Read the model definition and answer for the solid it produces. Units are mm, in the model's axes. A direction names the side the tool comes from. Round coordinates to 2 decimals unless told otherwise and drop trailing zeros. Loops run counter-clockwise (first coordinate to the right, second up) from the corner with the lowest first, then second, coordinate; pieces in that order, holes last. Notation, with made-up numbers: M -9,-13 L 19,-13 A27 cw 19,15 Z; hole C 73.5,7 d2. An arc over 180 degrees is marked long. Write each question's results on one line, items separated by ' | '.
from build123d import *

# Parameters (mm, degrees)
BULK_DEPTH              = 2.75
BULK_DEPTH_BACK         = 2.8
PEG_BASE_SKETCH_W       = 0.25
PEG_BASE_SKETCH_H       = 0.9
PEGS_DEPTH              = 3.35
RECEPTACLE_DEPTH        = 3.75
RECEPTACLE_DEPTH_BACK   = 0.75
SKETCH3_W               = 0.6
SKETCH3_H               = 0.4
UPPER_FINS_DEPTH        = 0.31
ALTIUM_AXIS_ALIGN_ANGLE = 90


with BuildPart() as part:
    # Base sketch → Bulk (new body, two sides)
    with BuildSketch(Plane.XY) as bulk_sk:
        Polygon((3.7, 2.35), (-3.7, 2.35), (-3.7, 0.896446609), (-2.803553391, 0), (2.803553391, 0), (3.7, 0.896446609), align=None)
    extrude(amount=BULK_DEPTH)
    extrude(bulk_sk.sketch, amount=-BULK_DEPTH_BACK)

    # Peg base sketch → Pegs (add)
    with BuildSketch(Plane(origin=(0, 2.35, 0), x_dir=(1, 0, 0), z_dir=(0, 1, 0))):
        with Locations((3.575, 0)):
            Rectangle(PEG_BASE_SKETCH_W, PEG_BASE_SKETCH_H)
        with Locations((-3.575, 0)):
            Rectangle(PEG_BASE_SKETCH_W, PEG_BASE_SKETCH_H)
    extrude(amount=-PEGS_DEPTH)

    # Base sketch<3> → Receptacle (cut, two sides)
    with BuildSketch(Plane.XY) as receptacle_sk:
        Polygon((-3.45, 1), (-2.7, 0.25), (2.7, 0.25), (3.45, 1), (3.45, 2.1), (-3.45, 2.1), align=None)
    extrude(amount=RECEPTACLE_DEPTH, mode=Mode.SUBTRACT)
    extrude(receptacle_sk.sketch, amount=-RECEPTACLE_DEPTH_BACK, mode=Mode.SUBTRACT)

    # Sketch3 → Upper fins (add)
    with BuildSketch(Plane(origin=(0, 2.35, 0), x_dir=(1, 0, 0), z_dir=(0, 1, 0))):
        with Locations((-2.375, -1.4)):
            Rectangle(SKETCH3_W, SKETCH3_H)
        with Locations((2.375, -1.4)):
            Rectangle(SKETCH3_W, SKETCH3_H)
    extrude(amount=UPPER_FINS_DEPTH)


with BuildPart() as part_1:
    # Altium axis align: moved
    add(part.part.rotate(Axis((0, 0, 0), (1, 0, 0)), ALTIUM_AXIS_ALIGN_ANGLE))


solid = part_1.part
Item 1: A flat-ended cylindrical pin translates along its axis: pin 1 (1 mm diameter, centred on x = 0, y = -1.5, fed in from -Z). Find the tip coordinate at first contact, or state that the pin passes through.
Outcome:
pin 1: stops at z = 0
Item 2: Straight lines are drawn through the part: line 1 (Z direction, x = 2.5, y = -1.4); line 2 (Z direction, x = 1.75, y = -0.25); line 3 (X direction, y = -1.4, z = 2.4) (3 decimals). For each, find the intervals that lie inside material, in ascending order.
Outcome:
line 1: z = 0 to 0.25, 2.1 to 2.66 | line 2: z = 0 to 0.25, 2.1 to 2.35 | line 3: x = -2.675 to -2.075, 2.075 to 2.675
Item 3: The part is cut by section A-A (y = -1.9). Determine the outline of the cut face in (x, z).
Outcome:
outline: M -3.7,0.9 L -2.8,0 L 2.8,0 L 3.7,0.9 L 3.7,2.35 L -3.7,2.35 Z; hole M -3.45,1 L -2.7,0.25 L 2.7,0.25 L 3.45,1 L 3.45,2.1 L -3.45,2.1 Z
Item 4: For faces 1 (the face through (0, -1, 2.1)), 2 (the face through (3.45, 0, 0)), 3 (the face through (3.7, 0, 1)), determine the directions among +Z, -Z, +X, -X, +Y, -Y from which every point of the face is accessible in a straight line to the end or side of a thin tool.
Outcome:
face 1: -Y | face 2: -Z, +Y, -Y | face 3: +Z, -Z, +X, +Y, -Y
Item 5: The part is cut by section D-D (z = 2). Determine the outline of the cut face in (x, y).
Outcome:
outline: M -3.7,-2.75 L -3.45,-2.75 L -3.45,0.75 L 3.45,0.75 L 3.45,-2.75 L 3.7,-2.75 L 3.7,2.8 L -3.7,2.8 Z
Item 6: The part is cut by section C-C (x = 2.25). Determine the outline of the cut face in (y, z), plus the area to 3 significant figures.
Outcome:
outline: M -2.75,0 L 2.8,0 L 2.8,2.35 L -1.2,2.35 L -1.2,2.66 L -1.6,2.66 L -1.6,2.35 L -2.75,2.35 L -2.75,2.1 L 0.75,2.1 L 0.75,0.25 L -2.75,0.25 Z | area: 6.69 mm2
Item 7: The part is cut by section B-B (z = 0.45). Determine the outline of the cut face in (x, y).
Outcome:
outline: M -3.7,-0.45 L -3.45,-0.45 L -3.45,0.45 L -3.7,0.45 Z; M -3.25,-2.75 L -2.9,-2.75 L -2.9,0.75 L 2.9,0.75 L 2.9,-2.75 L 3.25,-2.75 L 3.25,2.8 L -3.25,2.8 Z; M 3.45,-0.45 L 3.7,-0.45 L 3.7,0.45 L 3.45,0.45 Z
Item 8: The mould has two halves that part along X. Classify faces 4 (the face through (-3.7, 0, 1)), 5 (the face through (0, -1, 0.25)), 6 (the face through (0, 2.8, 1)): pulls with the +X half, pulls with the -X half, needs draft (parallel to the pull), parting line crosses it, or undercut.
Outcome:
face 4: pulls with the -X half | face 5: undercut | face 6: needs draft
